from build123d import *

# Parameters (mm, degrees)
BOSS_EXTRUDE1_DEPTH                              = 28.4
BOSS_EXTRUDE1_DEPTH_BACK                         = 4
SKETCH1_W                                        = 65.5
SKETCH1_H                                        = 65.5
SKETCH1_W_2                                      = 30.5
SKETCH1_H_2                                      = 35.6
CUT_EXTRUDE1_REACH                               = 98.887
SKETCH5_R                                        = 11.3
CUT_EXTRUDE4_REACH                               = 98.887
SKETCH7_R                                        = 5.3
SKETCH8_W                                        = 30.5
SKETCH8_H                                        = 35.6
BOSS_EXTRUDE2_DEPTH                              = 4
SKETCH9_R                                        = 4.9
CUT_EXTRUDE5_DEPTH                               = 2.2
FILLET1_R                                        = 2.5
CUT_EXTRUDE7_REACH                               = 98.887
SKETCH10_R                                       = 5
CBORE_FOR_M4_PAN_HEAD_MACHINE_SCREW1_D           = 4.8
CBORE_FOR_M4_PAN_HEAD_MACHINE_SCREW1_DEPTH       = 8
CBORE_FOR_M4_PAN_HEAD_MACHINE_SCREW1_CBORE_D     = 9
CBORE_FOR_M4_PAN_HEAD_MACHINE_SCREW1_CBORE_DEPTH = 3.1
CBORE_FOR_M4_PAN_HEAD_MACHINE_SCREW1_TIP         = 1.442065486
SKETCH23_W                                       = 112.7
SKETCH23_H                                       = 88
BOSS_EXTRUDE3_DEPTH                              = 3
SKETCH24_W                                       = 45
SKETCH24_H                                       = 4
BOSS_EXTRUDE4_DEPTH                              = 43.5
CBORE_FOR_M3_PAN_HEAD_MACHINE_SCREW1_D           = 3.2
CBORE_FOR_M3_PAN_HEAD_MACHINE_SCREW1_CBORE_D     = 7
CBORE_FOR_M3_PAN_HEAD_MACHINE_SCREW1_CBORE_DEPTH = 2.4
CUT_EXTRUDE8_REACH                               = 170.008
SKETCH28_R                                       = 12.5
SKETCH30_W                                       = 33.85
SKETCH30_H                                       = 30
BOSS_EXTRUDE5_DEPTH                              = 35
CUT_EXTRUDE10_REACH                              = 170.008
SKETCH31_R                                       = 4.25
CBORE_START                                      = -103.5
CBORE_FOR_M3_PAN_HEAD_MACHINE_SCREW2_OUT_R       = 3.5
CBORE_FOR_M3_PAN_HEAD_MACHINE_SCREW2_DEPTH       = 2.4
CBORE_START_2                                    = -101.1
CBORE_FOR_M3_PAN_HEAD_MACHINE_SCREW2_2_O_R       = 1.6
CBORE_FOR_M3_PAN_HEAD_MACHINE_SCREW2_2_DEPTH     = 4.162673424


# Read off the part's stored shape, not the designer's step: CBORE for M3 Pan Head Machine Screw2
with BuildPart() as part:
    # Sketch1 → Boss-Extrude1 (new, two sides: drawn at the far end of the back side and taken through both)
    with BuildSketch(Plane.XY.offset(-BOSS_EXTRUDE1_DEPTH_BACK)):
        with Locations((-32.75, -32.75)):
            Rectangle(SKETCH1_W, SKETCH1_H)
        with Locations((-32.75, -32.75)):
            Rectangle(SKETCH1_W_2, SKETCH1_H_2, mode=Mode.SUBTRACT)
    extrude(amount=BOSS_EXTRUDE1_DEPTH + BOSS_EXTRUDE1_DEPTH_BACK)

    # Sketch5 → Cut-Extrude1 (cut, up to next)
    with BuildSketch(Plane(origin=(0, 0, 0), x_dir=(0, 0, -1), z_dir=(1, 0, 0)), mode=Mode.PRIVATE) as cut_extrude1_sk1:
        with Locations((-15.05, -32.45)):
            Circle(SKETCH5_R)
    cut_extrude1_tool1 = extrude(cut_extrude1_sk1.sketch, amount=-CUT_EXTRUDE1_REACH, mode=Mode.PRIVATE) & part.part
    add(cut_extrude1_tool1.solids().sort_by_distance((0, -32.45, 15.05))[0], mode=Mode.SUBTRACT)

    # Sketch7 → Cut-Extrude4 (cut, up to next)
    with BuildSketch(Plane(origin=(-65.5, 0, 0), x_dir=(0, 0, -1), z_dir=(1, 0, 0)), mode=Mode.PRIVATE) as cut_extrude4_sk1:
        with Locations(Location((-15.05, -32.45, 0), (0, 0, 180))):
            Circle(SKETCH7_R)
    cut_extrude4_tool1 = extrude(cut_extrude4_sk1.sketch, amount=CUT_EXTRUDE4_REACH, mode=Mode.PRIVATE) & part.part
    add(cut_extrude4_tool1.solids().sort_by_distance((-65.5, -32.45, 15.05))[0], mode=Mode.SUBTRACT)

    # Sketch8 → Boss-Extrude2 (add)
    with BuildSketch(Plane(origin=(0, 0, -4), x_dir=(-1, 0, 0), z_dir=(0, 0, -1))):
        with Locations((32.75, -32.75)):
            Rectangle(SKETCH8_W, SKETCH8_H)
    extrude(amount=-BOSS_EXTRUDE2_DEPTH)

    # Sketch9 → Cut-Extrude5 (cut)
    with BuildSketch(Plane.XY.offset(-4)):
        with Locations((-12.75, -12.9)):
            Circle(SKETCH9_R)
        with Locations(Location((-52.75, -12.9, 0), (0, 0, 180))):
            Circle(SKETCH9_R)
        with Locations((-52.75, -52.6)):
            Circle(SKETCH9_R)
        with Locations(Location((-12.75, -52.6, 0), (0, 0, 180))):
            Circle(SKETCH9_R)
    extrude(amount=CUT_EXTRUDE5_DEPTH, mode=Mode.SUBTRACT)

    # Fillet1
    fillet1_edges = [part.edges().sort_by_distance(p)[0] for p in [
        (-65.5, 0, 12.2),
        (0, 0, 12.2),
    ]]
    fillet(fillet1_edges, radius=FILLET1_R)

    # Sketch10 → Cut-Extrude7 (cut, up to next)
    with BuildSketch(Plane.XY, mode=Mode.PRIVATE) as cut_extrude7_sk1:
        with Locations((-22.8, -12.9)):
            Circle(SKETCH10_R)
    cut_extrude7_tool1 = extrude(cut_extrude7_sk1.sketch, amount=CUT_EXTRUDE7_REACH, mode=Mode.PRIVATE) & part.part
    # Sketch10 → Cut-Extrude7 (cut, up to next)
    with BuildSketch(Plane.XY, mode=Mode.PRIVATE) as cut_extrude7_sk2:
        with Locations((-42.7, -12.9)):
            Circle(SKETCH10_R)
    cut_extrude7_tool2 = extrude(cut_extrude7_sk2.sketch, amount=CUT_EXTRUDE7_REACH, mode=Mode.PRIVATE) & part.part
    # Sketch10 → Cut-Extrude7 (cut, up to next)
    with BuildSketch(Plane.XY, mode=Mode.PRIVATE) as cut_extrude7_sk3:
        with Locations((-22.8, -52.6)):
            Circle(SKETCH10_R)
    cut_extrude7_tool3 = extrude(cut_extrude7_sk3.sketch, amount=CUT_EXTRUDE7_REACH, mode=Mode.PRIVATE) & part.part
    # Sketch10 → Cut-Extrude7 (cut, up to next)
    with BuildSketch(Plane.XY, mode=Mode.PRIVATE) as cut_extrude7_sk4:
        with Locations((-42.7, -52.6)):
            Circle(SKETCH10_R)
    cut_extrude7_tool4 = extrude(cut_extrude7_sk4.sketch, amount=CUT_EXTRUDE7_REACH, mode=Mode.PRIVATE) & part.part
    add(cut_extrude7_tool1.solids().sort_by_distance((-22.8, -12.9, 0))[0], mode=Mode.SUBTRACT)
    add(cut_extrude7_tool2.solids().sort_by_distance((-42.7, -12.9, 0))[0], mode=Mode.SUBTRACT)
    add(cut_extrude7_tool3.solids().sort_by_distance((-22.8, -52.6, 0))[0], mode=Mode.SUBTRACT)
    add(cut_extrude7_tool4.solids().sort_by_distance((-42.7, -52.6, 0))[0], mode=Mode.SUBTRACT)

    # CBORE for M4 Pan Head Machine Screw1
    with Locations(Plane(origin=(-42.7, -12.9, 0), x_dir=(1, 0, 0), z_dir=(0, 0, 1))):
        with Locations((0, 0), (19.9, 0), (0, -39.7), (19.9, -39.7)):
            CounterBoreHole(CBORE_FOR_M4_PAN_HEAD_MACHINE_SCREW1_D / 2, CBORE_FOR_M4_PAN_HEAD_MACHINE_SCREW1_CBORE_D / 2, CBORE_FOR_M4_PAN_HEAD_MACHINE_SCREW1_CBORE_DEPTH, depth=CBORE_FOR_M4_PAN_HEAD_MACHINE_SCREW1_DEPTH)
            with Locations((0, 0, -(CBORE_FOR_M4_PAN_HEAD_MACHINE_SCREW1_DEPTH + CBORE_FOR_M4_PAN_HEAD_MACHINE_SCREW1_TIP / 2))):  # 118° drill point
                Cone(0, CBORE_FOR_M4_PAN_HEAD_MACHINE_SCREW1_D / 2, CBORE_FOR_M4_PAN_HEAD_MACHINE_SCREW1_TIP, mode=Mode.SUBTRACT)

    # Sketch23 → Boss-Extrude3 (add)
    with BuildSketch(Plane.XZ.offset(65.5)):
        with Locations((-32.75, -15.6)):
            Rectangle(SKETCH23_W, SKETCH23_H)
    extrude(amount=BOSS_EXTRUDE3_DEPTH)

    # Sketch24 → Boss-Extrude4 (add)
    with BuildSketch(Plane(origin=(0, -68.5, 0), x_dir=(-1, 0, 0), z_dir=(0, -1, 0))):
        with Locations((32.75, -26.4)):
            Rectangle(SKETCH24_W, SKETCH24_H)
    extrude(amount=BOSS_EXTRUDE4_DEPTH)

    # CBORE for M3 Pan Head Machine Screw1 (through all)
    with Locations(Plane.XY.offset(28.4)):
        with Locations((-48.25, -74.5), (-48.25, -105.5)):
            cbore_for_m3_pan_head_machine_screw1 = CounterBoreHole(CBORE_FOR_M3_PAN_HEAD_MACHINE_SCREW1_D / 2, CBORE_FOR_M3_PAN_HEAD_MACHINE_SCREW1_CBORE_D / 2, CBORE_FOR_M3_PAN_HEAD_MACHINE_SCREW1_CBORE_DEPTH)

    # Sketch28 → Cut-Extrude8 (cut, up to next)
    with BuildSketch(Plane.XY.offset(28.4), mode=Mode.PRIVATE) as cut_extrude8_sk1:
        with Locations((-32.75, -90.25)):
            Circle(SKETCH28_R)
    cut_extrude8_tool1 = extrude(cut_extrude8_sk1.sketch, amount=-CUT_EXTRUDE8_REACH, mode=Mode.PRIVATE) & part.part
    add(cut_extrude8_tool1.solids().sort_by_distance((-32.75, -90.25, 28.4))[0], mode=Mode.SUBTRACT)

    # Mirror1: CBORE for M3 Pan Head Machine Screw1 across plane
    add(cbore_for_m3_pan_head_machine_screw1.mirror(Plane(origin=(-32.75, 0, 0), x_dir=(0, 0, 1), z_dir=(1, 0, 0))), mode=Mode.SUBTRACT)

    # Sketch30 → Boss-Extrude5 (add)
    with BuildSketch(Plane(origin=(0, -68.5, 0), x_dir=(-1, 0, 0), z_dir=(0, -1, 0))):
        with Locations((72.175, -13.4)):
            Rectangle(SKETCH30_W, SKETCH30_H)
    boss_extrude5 = extrude(amount=BOSS_EXTRUDE5_DEPTH)

    # Sketch31 → Cut-Extrude10 (cut, up to next)
    with BuildSketch(Plane.XY.offset(28.4), mode=Mode.PRIVATE) as cut_extrude10_sk1:
        with Locations((-72.75, -93)):
            Circle(SKETCH31_R)
    cut_extrude10_tool1 = extrude(cut_extrude10_sk1.sketch, amount=-CUT_EXTRUDE10_REACH, mode=Mode.PRIVATE) & part.part
    cut_extrude10 = cut_extrude10_tool1.solids().sort_by_distance((-72.75, -93, 28.4))[0]
    add(cut_extrude10, mode=Mode.SUBTRACT)

    # CBORE for M3 Pan Head Machine Screw2 out → CBORE for M3 Pan Head Machine Screw2 (cut)
    with BuildSketch(Plane(origin=(0, 0, 0), x_dir=(1, 0, 0), z_dir=(0, 1, 0)).offset(CBORE_START)):
        with Locations((-72.75, -13.4)):
            Circle(CBORE_FOR_M3_PAN_HEAD_MACHINE_SCREW2_OUT_R)
    cbore_for_m3_pan_head_machine_screw2 = extrude(amount=CBORE_FOR_M3_PAN_HEAD_MACHINE_SCREW2_DEPTH, mode=Mode.SUBTRACT)

    # CBORE for M3 Pan Head Machine Screw2 2 o → CBORE for M3 Pan Head Machine Screw2 2 (cut)
    with BuildSketch(Plane(origin=(0, 0, 0), x_dir=(1, 0, 0), z_dir=(0, 1, 0)).offset(CBORE_START_2)):
        with Locations((-72.75, -13.4)):
            Circle(CBORE_FOR_M3_PAN_HEAD_MACHINE_SCREW2_2_O_R)
    cbore_for_m3_pan_head_machine_screw2_2 = extrude(amount=CBORE_FOR_M3_PAN_HEAD_MACHINE_SCREW2_2_DEPTH, mode=Mode.SUBTRACT)

    # Mirror2: Boss-Extrude5, Cut-Extrude10, CBORE for M3 Pan Head Machine Screw2, CBORE for M3 Pan Head Machine Screw2 2 across plane
    add(boss_extrude5.mirror(Plane(origin=(-32.75, 0, 0), x_dir=(0, 0, 1), z_dir=(1, 0, 0))))
    add(cut_extrude10.mirror(Plane(origin=(-32.75, 0, 0), x_dir=(0, 0, 1), z_dir=(1, 0, 0))), mode=Mode.SUBTRACT)
    add(cbore_for_m3_pan_head_machine_screw2.mirror(Plane(origin=(-32.75, 0, 0), x_dir=(0, 0, 1), z_dir=(1, 0, 0))), mode=Mode.SUBTRACT)
    add(cbore_for_m3_pan_head_machine_screw2_2.mirror(Plane(origin=(-32.75, 0, 0), x_dir=(0, 0, 1), z_dir=(1, 0, 0))), mode=Mode.SUBTRACT)


solid = part.part
Design review of the part built by this model. Coordinates are the model's own, in mm. A direction names the side the tool comes from. Round coordinates to 2 decimals unless told otherwise and drop trailing zeros. Write each loop counter-clockwise with the first axis right and the second up, starting at its lowest first coordinate (ties: lowest second). Pieces come first, ordered by that corner, then holes.
Item 1: For faces 1 (the flat face through (-71, -101.1, 14)), 2 (the flat face through (-32, -112, 26)), 3 (the flat face through (-41, -15, -3.1)), 4 (the flat face through (-10.25, -86, 12)), 5 (the cylindrical face through (-56.872, -30.42, 19.946)), list the 3-axis set-ups (+Z, -Z, +X, -X, +Y, -Y) from which the entire face can be reached by the end or side of a thin tool; tool diameter is ignored.
Item 2: Consider section C-C on x = -42.7. Count the separate pieces of the cut face and the enclosed holes in it, and give its area (3 significant figures).
Item 3: Wall thickness on L1, parallel to Y at x = -32, z = 26; L2, parallel to Y at x = -17.25, z = 27.85; L3, parallel to Z at x = -72.75, y = -99.3: over which ranges is each line inside the solid? List them lowest first.
Item 4: Draft analysis for pull direction X (two halves, no side actions). For faces 6 (the cylindrical face through (-18.64, -54.32, -1.53)), 7 (the flat face through (0, -41, 5)), 8 (the cylindrical face through (-8.628, -21.246, 16.521)), state which applies: released by +X, released by -X, zero draft, split by the parting line, or undercut.
Item 5: Consider section D-D on y = -90.25. Give the boundary of the cut face in (x, z), and give its area (3 significant figures).
Item 6: Consider section A-A on y = -74.5. Give the boundary of the cut face in (x, z), and give its area (3 significant figures).
Item 7: For pin 1 Ø1 at (y, z) = (-44, 19) entering from +X; pin 2 Ø3 at (x, z) = (-74, -10.5) entering from -Y; pin 3 Ø2.5 at (x, y) = (-42, -53) entering from +Z; pin 4 Ø2 at (y, z) = (-105.5, 26.5) entering from -X, all flat-tipped, find the tip position at first contact; note any pin that passes through.
Item 8: Consider section B-B on x = -72.75. Give the boundary of the cut face in (y, z), and give its area (3 significant figures).
Check values:
1. face 1: -Y
1. face 2: +Z, -Z, +X, -X, -Y
1. face 3: +Z
1. face 4: -Z, -Y
1. face 5: +X, -X
2. separate pieces: 4
2. enclosed holes: 0
2. area: 1,020 mm2
3. L1: y = -112 to -102.73, -77.77 to -50.55, -14.95 to 0
3. L2: y = -112 to -109, -102 to -78, -71 to 0
3. L3: z = -1.6 to 11.8, 15 to 28.4
4. face 6: undercut
4. face 7: released by +X
4. face 8: zero draft
5. outline: (-89.1, -1.6) - (-75.99, -1.6) - (-75.99, 28.4) - (-89.1, 28.4) - close; (-69.51, -1.6) - (-55.25, -1.6) - (-55.25, 24.4) - (-45.25, 24.4) - (-45.25, 28.4) - (-69.51, 28.4) - close; (-20.25, 24.4) - (-10.25, 24.4) - (-10.25, -1.6) - (4.01, -1.6) - (4.01, 28.4) - (-20.25, 28.4) - close; (10.49, -1.6) - (23.6, -1.6) - (23.6, 28.4) - (10.49, 28.4) - close
5. area: 1,720 mm2
6. outline: (-89.1, -1.6) - (-55.25, -1.6) - (-55.25, 24.4) - (-49.85, 24.4) - (-49.85, 26) - (-51.75, 26) - (-51.75, 28.4) - (-89.1, 28.4) - close; (-46.65, 24.4) - (-18.85, 24.4) - (-18.85, 26) - (-20.75, 26) - (-20.75, 28.4) - (-44.75, 28.4) - (-44.75, 26) - (-46.65, 26) - close; (-15.65, 24.4) - (-10.25, 24.4) - (-10.25, -1.6) - (23.6, -1.6) - (23.6, 28.4) - (-13.75, 28.4) - (-13.75, 26) - (-15.65, 26) - close
6. area: 2,170 mm2
7. pin 1: stops at x = 0
7. pin 2: stops at y = -68.5
7. pin 3: passes through
7. pin 4: stops at x = -55.25
8. outline: (-103.5, -1.6) - (-97.25, -1.6) - (-97.25, 11.8) - (-101.1, 11.8) - (-101.1, 9.9) - (-103.5, 9.9) - close; (-103.5, 16.9) - (-101.1, 16.9) - (-101.1, 15) - (-97.25, 15) - (-97.25, 28.4) - (-103.5, 28.4) - close; (-88.75, -1.6) - (-68.5, -1.6) - (-68.5, -59.6) - (-65.5, -59.6) - (-65.5, 28.4) - (-88.75, 28.4) - close
8. area: 1,030 mm2
